Can you work these out from the model? Positions are in its coordinate system, mm. A direction names the side the tool comes from. Coordinates: 2 decimals unless noted, no trailing zeros. Order: outer loops, then holes, each group sorted by start corner. A loop starts at its lowest first (then second) coordinate and runs counter-clockwise, first axis right, second up. Notation, with made-up numbers: M 6.25,1 L 43.25,1 A28 cw 43.25,34 Z; hole C 23,35.25 d5. An arc over 180 degrees is marked long. Answer as a JSON object with one key per item and string values.
from build123d import *

# Parameters (mm, degrees)
F0_W     = 85
F0_H     = 23
F1_DEPTH = 3
F2_W     = 3
F2_H     = 23
F3_DEPTH = 24
F4_W     = 3
F4_H     = 23
F5_DEPTH = 25
F6_R     = 4
F6_R_2   = 2
F7_DEPTH = 100
F8_R     = 5


with BuildPart() as f1:
    # F0 (on Top) → F1 (new body)
    with BuildSketch(Plane.XY):
        with Locations((42.5, 11.5)):
            Rectangle(F0_W, F0_H)
        with BuildLine():
            Line((85, 0), (0, 0))
            Line((0, 0), (0, -10))
            Line((0, -10), (0, -65))
            ThreePointArc((0, -65), (1.464466, -68.535534), (5, -70))
            Line((5, -70), (7.5, -70))
            ThreePointArc((7.5, -70), (11.035534, -68.535534), (12.5, -65))
            Line((12.5, -65), (12.5, -15))
            ThreePointArc((12.5, -15), (13.964466, -11.464466), (17.5, -10))
            Line((17.5, -10), (67.5, -10))
            ThreePointArc((67.5, -10), (71.035534, -11.464466), (72.5, -15))
            Line((72.5, -15), (72.5, -65))
            ThreePointArc((72.5, -65), (73.964466, -68.535534), (77.5, -70))
            Line((77.5, -70), (80, -70))
            ThreePointArc((80, -70), (83.535534, -68.535534), (85, -65))
            Line((85, -65), (85, -10))
            Line((85, -10), (85, 0))
        make_face()
    extrude(amount=F1_DEPTH)

    # F2 (on face) → F3 (join)
    with BuildSketch(Plane.XY.offset(3)):
        with Locations((1.5, 11.5)):
            Rectangle(F2_W, F2_H)
        with Locations((83.5, 11.5)):
            Rectangle(F2_W, F2_H)
    extrude(amount=F3_DEPTH)

    # F4 (on face) → F5 (join)
    with BuildSketch(Plane.XY.offset(27)):
        with Locations((1.5, 11.5)):
            Rectangle(F4_W, F4_H)
    extrude(amount=F5_DEPTH)

    # F6 (on face) → F7 (cut)
    with BuildSketch(Plane.YZ.offset(85)):
        with Locations((11.5, 13.5)):
            Circle(F6_R)
        with Locations((19.5, 13.5)):
            Circle(F6_R_2)
        with Locations((11.5, 21.5)):
            Circle(F6_R_2)
        with Locations((3.5, 13.5)):
            Circle(F6_R_2)
        with Locations((11.5, 5.5)):
            Circle(F6_R_2)
    extrude(amount=-F7_DEPTH, mode=Mode.SUBTRACT)

    # F8
    f8_edges = [f1.edges().sort_by_distance(p)[0] for p in [
        (83.5, 0, 27),
        (83.5, 23, 27),
        (1.5, 23, 52),
        (1.5, 0, 52),
    ]]
    fillet(f8_edges, radius=F8_R)


solid = f1.part
Item 1: I want a section at C-C, the plane z = 13.5. Give the number of separate pieces and of enclosed holes in the cut face, plus the area to 3 significant figures.
Answers follow:
{"separate pieces": "8", "enclosed holes": "0", "area": "42.0 mm^2"}
Item 2: Please list where these lines run through material, in increasing order: line 1 (Z direction, x = 83.45, y = 11.5); line 2 (Z direction, x = 25, y = 14); line 3 (Y direction, x = 84, z = 13).
Answers follow:
{"line 1": "z = 0 to 3.5, 7.5 to 9.5, 17.5 to 19.5, 23.5 to 27", "line 2": "z = 0 to 3", "line 3": "y = 0 to 1.56, 5.44 to 7.53, 15.47 to 17.56, 21.44 to 23"}
Item 3: Which directions (+Z, -Z, +X, -X, +Y, -Y) give clear straight access to the entire face, cutting with the end or side of a thin tool? Please do faces 4 (the cylindrical face through (11, -68.57, 1.48)), 5 (the flat face through (3, 11, 27)), 6 (the cylindrical face through (84, 22, 25)), 7 (the cylindrical face through (84, 2, 26)).
Answers follow:
{"face 4": "+Z, -Z, -Y", "face 5": "+Z, +Y, -Y", "face 6": "+Z, +X, +Y", "face 7": "+Z, +X, -Y"}
Item 4: If we mould it in two halves opening along X, with no side actions, what happens to faces 1 (the flat face through (83, 12, 27)), 2 (the flat face through (82, 14, 17)), 3 (the flat face through (0, 2, 24))? For each: pulls with the +X half, pulls with the -X half, needs draft (parallel to the pull), parting line crosses it, or undercut.
Answers follow:
{"face 1": "needs draft", "face 2": "undercut", "face 3": "pulls with the -X half"}
Item 5: I want a section at B-B, the plane y = -50. Write out the boundary of the cut face in (x, z).
Answers follow:
{"outline": "M 0,0 L 12.5,0 L 12.5,3 L 0,3 Z; M 72.5,0 L 85,0 L 85,3 L 72.5,3 Z"}
Item 6: I'm going to push flat-ended pins straight in: pin 1 (6.5 mm diameter, centred on y = 19.5, z = 13.5, fed in from -X); pin 2 (2.5 mm diameter, centred on x = 83, y = 13.5, fed in from +Z); pin 3 (2.5 mm diameter, centred on x = 84, z = 9, fed in from -Y); pin 4 (0.9 mm diameter, centred on x = 36.5, z = 1.5, fed in from -Y). Where does each tip first touch, or does it pass through?
Answers follow:
{"pin 1": "stops at x = 0", "pin 2": "stops at z = 27", "pin 3": "stops at y = 0", "pin 4": "stops at y = -10"}
Item 7: I want a section at A-A, the plane z = 25. Write out the boundary of the cut face in (x, y).
Answers follow:
{"outline": "M 0,0 L 3,0 L 3,23 L 0,23 Z; M 82,1 L 85,1 L 85,22 L 82,22 Z"}
